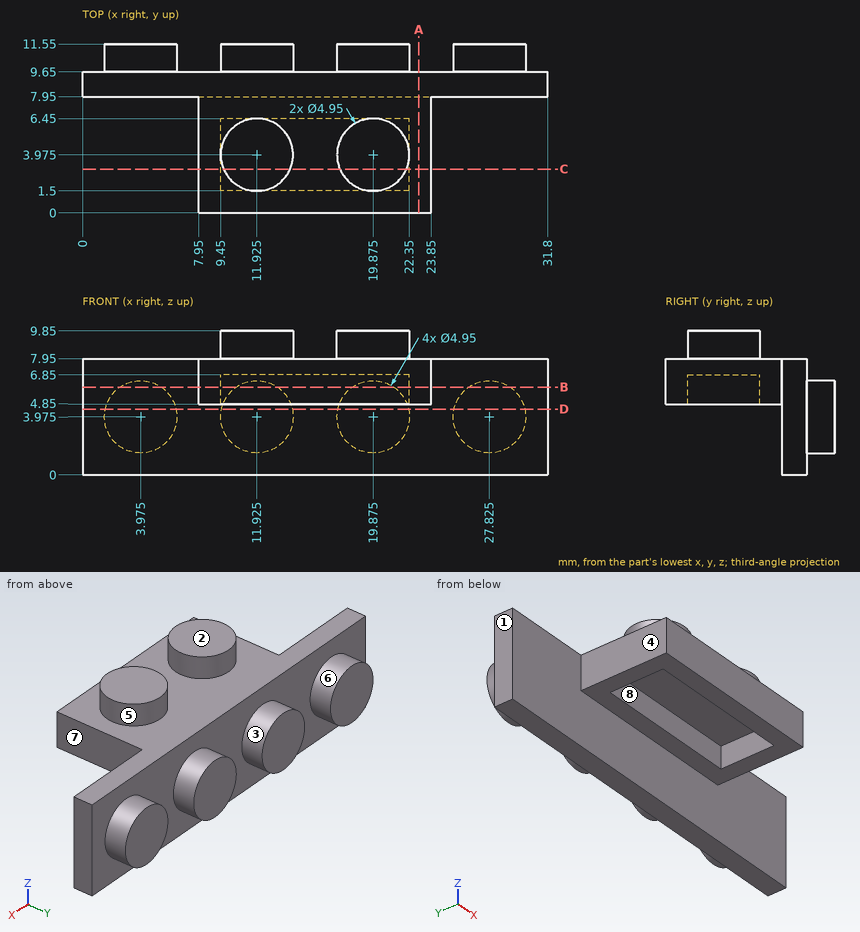
Job drawing, mm, ordinate dimensions from the low corner. One solid piece. A direction names the side the tool comes from. Give positions to 0.01 mm unless a question says otherwise; leave off trailing zeros. Loops run counter-clockwise (first coordinate to the right, second up) from the corner with the lowest first, then second, coordinate; pieces in that order, holes last. Notation, with made-up numbers: (21.5, 32.5) -> (61.5, 32.5) arc R25 ccw to (61.5, 53.5) -> close; hole circle Ø2 at (2, 53). An arc over 180 degrees is marked (long way). Use a Markdown table: item, result. Add a question column.
(1) Slice it at D-D on z = 4.5. List the corners of the cut face in (x, y).
(2) Mould opens along X. For the marked faces 1, 2 and 3 say: +X half, -X half, draft (parallel to the pull), parting line (faces both ways), or undercut.
(3) Wall check: line 1 along X through (y, z) = (5, 5.75); line 2 along Y through (x, z) = (19.5, 5.5); line 3 along Y through (x, z) = (29.5, 1.5). Give the ranges that are in metal, low to high.
(4) Slice it at C-C on y = 3. List the corners of the cut face in (x, z).
(5) Tool access for the marked faces 4, 5, 6, 7 and 8: list every direction of +Z, -Z, +X, -X, +Y, -Y with a clear straight run to the whole face (end or side of a thin tool).
(6) Slice it at B-B on z = 6. List the corners of the cut face in (x, y).
(7) Drop flat-ended pins along their axis: pin 1 Ø1.5 at (y, z) = (2.5, 6) entering from +X; pin 2 Ø3 at (x, y) = (13, 9.5) entering from +Z; pin 3 Ø2 at (x, z) = (18.5, 3) entering from -Y. Give the stop position or say it passes through.
(8) Slice it at A-A on x = 23. List the corners of the cut face in (y, z).
Filled sheet:
| question | item | result |
|---|---|---|
| 1 | outline | (0, 7.95) -> (31.8, 7.95) -> (31.8, 9.65) -> (30.24, 9.65) -> (30.24, 11.55) -> (25.41, 11.55) -> (25.41, 9.65) -> (22.29, 9.65) -> (22.29, 11.55) -> (17.46, 11.55) -> (17.46, 9.65) -> (14.34, 9.65) -> (14.34, 11.55) -> (9.51, 11.55) -> (9.51, 9.65) -> (6.39, 9.65) -> (6.39, 11.55) -> (1.56, 11.55) -> (1.56, 9.65) -> (0, 9.65) -> close |
| 2 | face 1 | -X half |
| 2 | face 2 | draft |
| 2 | face 3 | undercut |
| 3 | line 1 | 7.95 to 9.45, 22.35 to 23.85 |
| 3 | line 2 | 0 to 1.5, 6.45 to 11.55 |
| 3 | line 3 | 7.95 to 9.65 |
| 4 | outline | (7.95, 4.85) -> (9.45, 4.85) -> (9.45, 6.85) -> (22.35, 6.85) -> (22.35, 4.85) -> (23.85, 4.85) -> (23.85, 7.95) -> (22.15, 7.95) -> (22.15, 9.85) -> (17.6, 9.85) -> (17.6, 7.95) -> (14.2, 7.95) -> (14.2, 9.85) -> (9.65, 9.85) -> (9.65, 7.95) -> (7.95, 7.95) -> close |
| 5 | face 4 | +Z, -Z, -X, -Y |
| 5 | face 5 | +Z |
| 5 | face 6 | +Y |
| 5 | face 7 | +Z, -Z, +X, -Y |
| 5 | face 8 | -Z |
| 6 | outline | (0, 7.95) -> (7.95, 7.95) -> (7.95, 0) -> (23.85, 0) -> (23.85, 7.95) -> (31.8, 7.95) -> (31.8, 9.65) -> (29.25, 9.65) -> (29.25, 11.55) -> (26.4, 11.55) -> (26.4, 9.65) -> (21.3, 9.65) -> (21.3, 11.55) -> (18.45, 11.55) -> (18.45, 9.65) -> (13.35, 9.65) -> (13.35, 11.55) -> (10.5, 11.55) -> (10.5, 9.65) -> (5.4, 9.65) -> (5.4, 11.55) -> (2.55, 11.55) -> (2.55, 9.65) -> (0, 9.65) -> close; hole (9.45, 1.5) -> (22.35, 1.5) -> (22.35, 6.45) -> (9.45, 6.45) -> close |
| 7 | pin 1 | x = 23.85 |
| 7 | pin 2 | z = 7.95 |
| 7 | pin 3 | y = 7.95 |
| 8 | outline | (0, 4.85) -> (7.95, 4.85) -> (7.95, 0) -> (9.65, 0) -> (9.65, 7.95) -> (0, 7.95) -> close |
